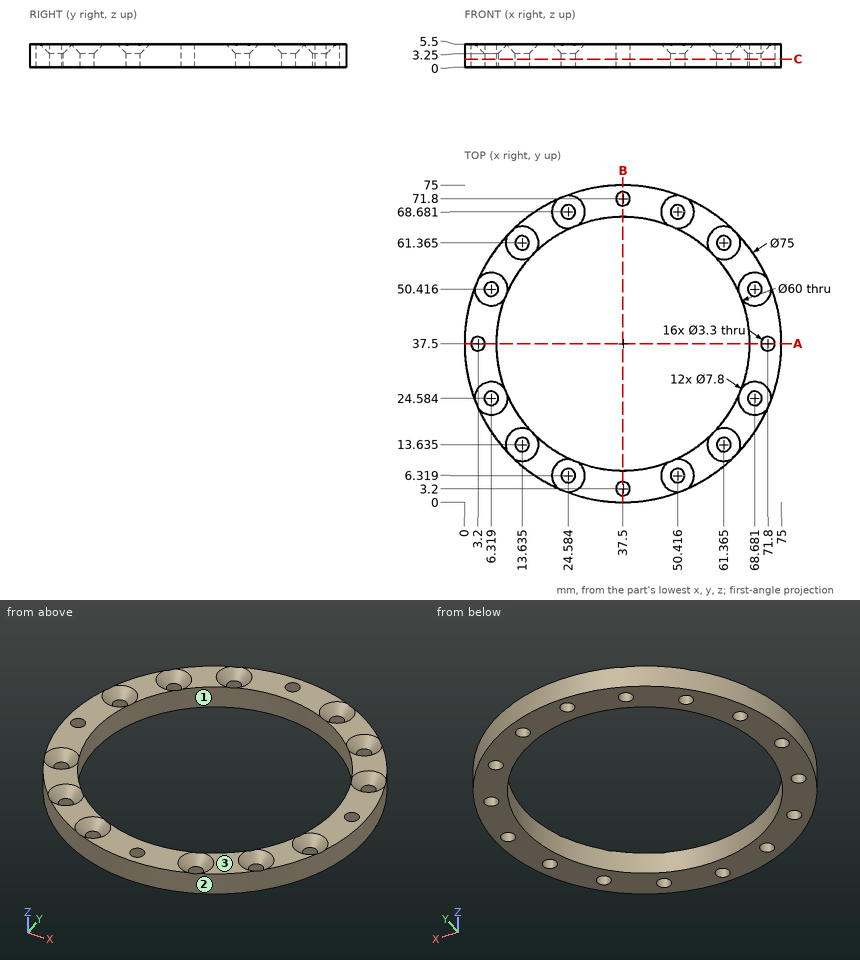
For this review, use the dimensioned drawing (mm, ordinates from the lowest corner) and the shaded views. Give positions to 0.01 mm unless a question says otherwise; leave off trailing zeros. Write each loop counter-clockwise with the first axis right and the second up, starting at its lowest first coordinate (ties: lowest second). Pieces come first, ordered by that corner, then holes. Notation, with made-up numbers: M 19.5,-25 L 38.5,-25 A20 cw 38.5,-15 Z; hole C 85.5,57.25 d1. An arc over 180 degrees is marked long. Answer as a JSON object with one key per item and string values. Group by question number.
Item 1: For pin 1 Ø4 at (x, y) = (61.36, 61.36) entering from -Z; pin 2 Ø2.5 at (x, y) = (37.5, 3.2) entering from -Z; pin 3 Ø1 at (y, z) = (58, 4) entering from -X; pin 4 Ø2 at (y, z) = (26.5, 4) entering from +X, all flat-tipped, find the tip position at first contact; note any pin that passes through.
Item 2: Draft analysis for pull direction X (two halves, no side actions). For the marked faces 1, 2 and 3, state which applies: +X half, -X half, draft (parallel to the pull), parting line (faces both ways), or undercut.
Item 3: Consider section C-C on z = 1.9. Count the separate pieces of the cut face and the enclosed holes in it, plus the area to 3 significant figures.
Item 4: Consider section A-A on y = 37.5. Write out the cut boundary in (x, z).
Item 5: For probe 1 along Y at (x, z) = (37.5, 4.25); probe 2 along X at (y, z) = (24, 4.95) (1 decimal); probe 3 along X at (y, z) = (39, 2.05) (1 decimal), list the stretches that pass through material, from the lowest coordinate up. Write a range as [from, to].
Check result:
{
 "1": {"pin 1": "stops at z = 0", "pin 2": "passes through", "pin 3": "stops at x = 5.78", "pin 4": "stops at x = 73.64"},
 "2": {"face 1": "undercut", "face 2": "parting line", "face 3": "draft"},
 "3": {"separate pieces": "1", "enclosed holes": "17", "area": "1,450 mm^2"},
 "4": {"outline": "M 0,0 L 1.55,0 L 1.55,5.5 L 0,5.5 Z; M 4.85,0 L 7.5,0 L 7.5,5.5 L 4.85,5.5 Z; M 67.5,0 L 70.15,0 L 70.15,5.5 L 67.5,5.5 Z; M 73.45,0 L 75,0 L 75,5.5 L 73.45,5.5 Z"},
 "5": {"probe 1": "y = [0, 1.55], [4.85, 7.5], [67.5, 70.15], [73.45, 75]", "probe 2": "x = [2.5, 3], [9.6, 10.7], [64.3, 65.4], [72, 72.5]", "probe 3": "x = [0, 2.5], [3.9, 7.5], [67.5, 71.1], [72.5, 75]"}
}
